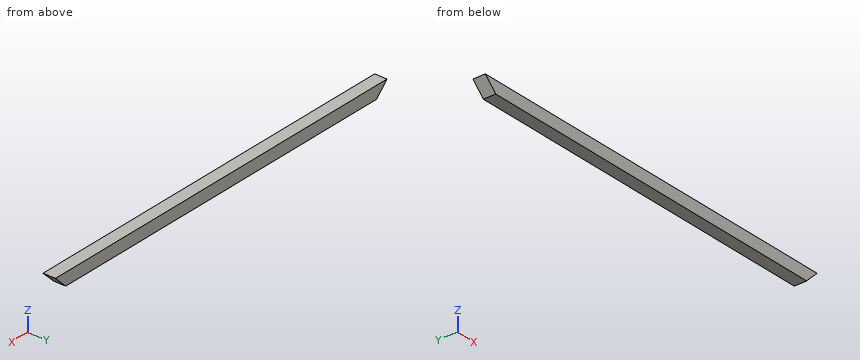
```python
from build123d import *

# Parameters (mm, degrees)
F0_W          = 25
F0_H          = 25
F1_DEPTH      = 800
F3_DEPTH      = 12.501
F3_DEPTH_BACK = 12.501
F5_DEPTH      = 12.501
F5_DEPTH_BACK = 12.501


with BuildPart() as f1:
    # F0 (on Right) → F1 (new body)
    with BuildSketch(Plane.YZ):
        Rectangle(F0_W, F0_H)
    extrude(amount=F1_DEPTH)

    # F2 (on Front) → F3 (cut, two sides)
    with BuildSketch(Plane.XZ) as f3_sk:
        Polygon((25, -12.5), (0, 12.5), (0, -12.5), align=None)
    extrude(amount=-F3_DEPTH, mode=Mode.SUBTRACT)
    extrude(f3_sk.sketch, amount=F3_DEPTH_BACK, mode=Mode.SUBTRACT)

    # F4 (on Front) → F5 (cut, two sides)
    with BuildSketch(Plane.XZ) as f5_sk:
        Polygon((800, -12.5), (800, 12.5), (775, -12.5), align=None)
    extrude(amount=-F5_DEPTH, mode=Mode.SUBTRACT)
    extrude(f5_sk.sketch, amount=F5_DEPTH_BACK, mode=Mode.SUBTRACT)


solid = f1.part
```
Verification items for the finished model (mm, model axes). Round coordinates to 2 decimals unless told otherwise and drop trailing zeros. Write each loop counter-clockwise with the first axis right and the second up, starting at its lowest first coordinate (ties: lowest second). Pieces come first, ordered by that corner, then holes. Notation, with made-up numbers: (67.5, 52) -> (126.5, 52) arc R30 cw to (126.5, 89) -> close; hole circle Ø2 at (35.5, 83.5). An arc over 180 degrees is marked (long way). Write each question's results on one line, items separated by ' | '. Start each with the question number.
1. Cross-section at A-A (z = 1.25). Enter the section's corners in (x, y).
2. Cross-section at B-B (y = -6.25). Enter the section's corners in (x, z), then the cut area to 3 significant figures.
3. Material ranges on probe 1 along X at (y, z) = (4.25, -6.75); probe 2 along X at (y, z) = (8.25, 11.25), recorded low to high. Write a range as from..to.
4. Depth check by flat-ended pin: P1, Ø1.5, axis at y = 4, z = -3, coming from the +X side; P2, Ø3, axis at y = -9.5, z = 1.5, coming from the -X side; P3, Ø5, axis at y = -10, z = 7, coming from the -X side. Enter the tip coordinate at first touch or a pass-through.
Solutions:
1) outline: (11.25, -12.5) -> (788.75, -12.5) -> (788.75, 12.5) -> (11.25, 12.5) -> close
2) outline: (0, 12.5) -> (25, -12.5) -> (775, -12.5) -> (800, 12.5) -> close | area: 19,400 mm2
3) probe 1: x = 19.25..780.75 | probe 2: x = 1.25..798.75
4) P1: stops at x = 785.25 | P2: stops at x = 9.5 | P3: stops at x = 3
